Model file for the job. Use its own axes, mm. A direction names the side the tool comes from. Round coordinates to 2 decimals unless told otherwise and drop trailing zeros. Order: outer loops, then holes, each group sorted by start corner. A loop starts at its lowest first (then second) coordinate and runs counter-clockwise, first axis right, second up. Notation, with made-up numbers: (32.5, 4.25) -> (37.5, 4.25) arc R22 cw to (37.5, 40.25) -> close; hole circle Ø10 at (34, 46). An arc over 180 degrees is marked (long way). Answer as CSV lines item,"result".
```python
from build123d import *

# Parameters (mm, degrees)
F1_DEPTH     = 3.175
F3_W         = 1562.1
F3_H         = 50.8
F4_DEPTH     = 3.175
F5_T         = 2.54
F5_T3_DEPTH  = 8.255
F5_T5_DEPTH  = 1567.18
F6_T         = 2.54
F6_T3_DEPTH  = 8.255
F6_T5_DEPTH  = 8.255
F6_T7_DEPTH  = 1567.18
F6_T9_DEPTH  = 5.715
F6_T11_DEPTH = 50.165
F6_T13_DEPTH = 5.715
F6_T15_DEPTH = 1562.1


# Not quite as in the source:
# - a shell that OpenCascade refuses in one call is made with other operations: the cavity is built on its own and cut out


with BuildPart() as f1:
    # F0 (on Front) → F1 (new body)
    with BuildSketch(Plane.XZ):
        Polygon((-781.05, 156.1854919385), (-793.75, 156.1854919385), (-793.75, 3.7854919385), (793.75, 3.7854919385), (793.75, 156.1854919385), (781.05, 156.1854919385), (781.05, 35.5354919385), (-781.05, 35.5354919385), align=None)
    extrude(amount=F1_DEPTH)

    # F3 (on face) → F4 (join)
    with BuildSketch(Plane.XY.offset(35.5354919385)):
        with Locations((0, 22.225)):
            Rectangle(F3_W, F3_H)
    extrude(amount=-F4_DEPTH)

    # F5: shell of thickness 2.54, made by hand


with BuildPart() as f5_core1:
    # F5_t2: copy of F1
    add(f1.part)

    # the walls: a layer under each face that stays
    f5_faces = [f5_core1.faces().sort_by_distance(p)[0] for p in [
        (-781.05, -1.5875, 95.8604919385),
        (-787.4, -1.5875, 156.1854919385),
        (-529.1666666667, 0, 29.1854919385),
        (-529.1666666667, -3.175, 29.1854919385),
        (781.05, -1.5875, 95.8604919385),
        (-793.75, -1.5875, 79.9854919385),
        (-781.05, 23.8125, 33.9479919385),
        (0, 23.8125, 32.3604919385),
        (781.05, 23.8125, 33.9479919385),
        (787.4, -1.5875, 156.1854919385),
        (793.75, -1.5875, 79.9854919385),
        (0, -1.5875, 3.7854919385),
        (0, 47.625, 33.9479919385),
    ]]
    thicken(f5_faces, amount=-F5_T, mode=Mode.SUBTRACT)

    # F5_s4 → F5_t3 (cut)
    with BuildSketch(Plane.XY.offset(29.8204919385)):
        Polygon((-781.0754, 0.0254), (-781.05, -2.54), (-778.51, -2.54), (-778.51, 0), align=None)
        Polygon((781.0754, 0.0254), (781.05, -2.54), (778.51, -2.54), (778.51, 0), align=None)
    extrude(amount=F5_T3_DEPTH, mode=Mode.SUBTRACT)

    # F5_s6 → F5_t5 (cut)
    with BuildSketch(Plane.YZ.offset(-783.59)):
        Polygon((0.0254, 32.3350919385), (-2.54, 32.3604919385), (-2.54, 34.9004919385), (0, 34.9004919385), align=None)
    extrude(amount=F5_T5_DEPTH, mode=Mode.SUBTRACT)


with BuildPart() as f1_1:
    add(f1.part)

    # what is left inside the walls is the cavity
    f5_cavity = [f5_core1.part.solids().sort_by_distance(p)[0] for p in [
        (0, 14.605, 34.925892),
    ]]
    add(f5_cavity, mode=Mode.SUBTRACT)

    # F6: shell of thickness 2.54, made by hand


with BuildPart() as f6_core1:
    # F6_t2: copy of F1
    add(f1_1.part)

    # the walls: a layer under each face that stays
    f6_faces = [f6_core1.faces().sort_by_distance(p)[0] for p in [
        (-781.05, -1.5875, 95.8604919385),
        (728.98, -1.4816666667, 35.5354919385),
        (-787.4, -1.5875, 156.1854919385),
        (-529.1666666667, 0, 29.1854919385),
        (781.05, -1.5875, 95.8604919385),
        (781.05, 23.8125, 33.9479919385),
        (0, 47.625, 33.9479919385),
        (-781.05, 23.8125, 33.9479919385),
        (778.51, 22.225, 35.2179919385),
        (0, -0.635, 35.2179919385),
        (-778.51, 22.225, 35.2179919385),
        (0, 45.085, 35.2179919385),
        (-793.75, -1.5875, 79.9854919385),
        (0, 23.8125, 32.3604919385),
        (787.4, -1.5875, 156.1854919385),
        (793.75, -1.5875, 79.9854919385),
        (0, -1.5875, 3.7854919385),
        (0, 22.225, 34.9004919385),
    ]]
    thicken(f6_faces, amount=-F6_T, mode=Mode.SUBTRACT)

    # F6_s4 → F6_t3 (cut)
    with BuildSketch(Plane.XZ.offset(-2.54)):
        Polygon((-781.0246, 35.5608919385), (-783.59, 35.5354919385), (-783.59, 32.9954919385), (-781.05, 32.9954919385), align=None)
        Polygon((781.0246, 35.5608919385), (781.05, 32.9954919385), (783.59, 32.9954919385), (783.59, 35.5354919385), align=None)
    extrude(amount=F6_T3_DEPTH, mode=Mode.SUBTRACT)

    # F6_s6 → F6_t5 (cut)
    with BuildSketch(Plane.XY.offset(29.8204919385)):
        Polygon((-781.0754, 0.0254), (-781.05, -2.54), (-778.51, -2.54), (-778.51, 0), align=None)
        Polygon((781.0754, 0.0254), (781.05, -2.54), (778.51, -2.54), (778.51, 0), align=None)
    extrude(amount=F6_T5_DEPTH, mode=Mode.SUBTRACT)

    # F6_s8 → F6_t7 (cut)
    with BuildSketch(Plane.YZ.offset(-783.59)):
        Polygon((0.0254, 32.3350919385), (-2.54, 32.3604919385), (-2.54, 34.9004919385), (0, 34.9004919385), align=None)
    extrude(amount=F6_T7_DEPTH, mode=Mode.SUBTRACT)

    # F6_s10 → F6_t9 (cut)
    with BuildSketch(Plane.XY.offset(32.3604919385)):
        Polygon((778.4846, 45.0596), (781.05, 45.085), (781.05, 47.625), (778.51, 47.625), align=None)
        Polygon((778.4846, -0.6096), (781.05, -0.635), (781.05, -3.175), (778.51, -3.175), align=None)
        Polygon((-778.4846, -0.6096), (-778.51, -3.175), (-781.05, -3.175), (-781.05, -0.635), align=None)
        Polygon((-778.4846, 45.0596), (-781.05, 45.085), (-781.05, 47.625), (-778.51, 47.625), align=None)
    extrude(amount=F6_T9_DEPTH, mode=Mode.SUBTRACT)

    # F6_s12 → F6_t11 (cut)
    with BuildSketch(Plane.XZ.offset(-47.625)):
        Polygon((778.4846, 34.9258919385), (781.05, 34.9004919385), (781.05, 32.3604919385), (778.51, 32.3604919385), align=None)
        Polygon((-778.4846, 34.9258919385), (-781.05, 34.9004919385), (-781.05, 32.3604919385), (-778.51, 32.3604919385), align=None)
    extrude(amount=F6_T11_DEPTH, mode=Mode.SUBTRACT)

    # F6_s14 → F6_t13 (cut)
    with BuildSketch(Plane.XZ.offset(-2.54)):
        Polygon((778.4846, 34.9258919385), (781.05, 34.9004919385), (781.05, 32.3604919385), (778.51, 32.3604919385), align=None)
        Polygon((-778.4846, 34.9258919385), (-781.05, 34.9004919385), (-781.05, 32.3604919385), (-778.51, 32.3604919385), align=None)
    extrude(amount=F6_T13_DEPTH, mode=Mode.SUBTRACT)

    # F6_s16 → F6_t15 (cut)
    with BuildSketch(Plane.YZ.offset(-781.05)):
        Polygon((-0.6096, 34.9258919385), (-3.175, 34.9004919385), (-3.175, 32.3604919385), (-0.635, 32.3604919385), align=None)
        Polygon((45.0596, 34.9258919385), (47.625, 34.9004919385), (47.625, 32.3604919385), (45.085, 32.3604919385), align=None)
    extrude(amount=F6_T15_DEPTH, mode=Mode.SUBTRACT)


with BuildPart() as f1_2:
    add(f1_1.part)

    # what is left inside the walls is the cavity
    f6_cavity = [f6_core1.part.solids().sort_by_distance(p)[0] for p in [
        (395.605, -2.5654, 22.694381),
    ]]
    add(f6_cavity, mode=Mode.SUBTRACT)


solid = f1_2.part
```
Q1. Flat gauge pins, fed straight in: pin 1 (3 mm diameter, centred on x = -313, y = 5.5, fed in from +Z); pin 2 (1.6 mm diameter, centred on y = 14.5, z = 33.5, fed in from +X); pin 3 (0.5 mm diameter, centred on x = -103, y = -3, fed in from +Z). Where does each tip first touch, or does it go through?
Checks:
pin 1,"z = 34.9"
pin 2,"x = 781.05"
pin 3,"z = 35.54"
Q2. Saw through at C-C (x = 440). Write the cut outline in (y, z) (1 decimal).
Checks:
outline,"(-3.2, 3.8) -> (0, 3.8) -> (0, 32.4) -> (47.6, 32.4) -> (47.6, 35.5) -> (45.1, 35.5) -> (45.1, 34.9) -> (-0.6, 34.9) -> (-0.6, 35.5) -> (-3.2, 35.5) -> (-3.2, 32.4) -> (-2.5, 32.4) -> (-2.5, 6.3) -> (-3.2, 6.3) -> close"
Q3. Wall check: L1, parallel to Z at x = -432, y = 21. Give the ranges that are in metal, low to high. Write a range as [from, to].
Checks:
L1,"[32.36, 34.9]"
Q4. Tool access for faces 1 (the flat face through (-11, 24, 32.36)), 2 (the flat face through (4, -2, 35.535)), 3 (the flat face through (-4, -3.175, 35)): list every direction of +Z, -Z, +X, -X, +Y, -Y with a clear straight run to the whole face (end or side of a thin tool).
Checks:
face 1,"-Z, +X, -X, +Y"
face 2,"+Z, +Y, -Y"
face 3,"+Z, -Z, +X, -X, -Y"
Q5. Saw through at A-A (z = 106). Write the cut outline in (x, y) (3 decimals).
Checks:
outline,"(-793.75, -3.175) -> (-791.21, -3.175) -> (-791.21, -2.54) -> (-783.59, -2.54) -> (-783.59, -3.175) -> (-781.05, -3.175) -> (-781.05, 0) -> (-793.75, 0) -> close; (781.05, -3.175) -> (783.59, -3.175) -> (783.59, -2.54) -> (791.21, -2.54) -> (791.21, -3.175) -> (793.75, -3.175) -> (793.75, 0) -> (781.05, 0) -> close"
Q6. Saw through at B-B (y = 8.5). Write the cut outline in (x, z), plus the area to 3 significant figures.
Checks:
outline,"(-781.05, 32.36) -> (781.05, 32.36) -> (781.05, 35.54) -> (778.51, 35.54) -> (778.51, 34.9) -> (-778.51, 34.9) -> (-778.51, 35.54) -> (-781.05, 35.54) -> close"
area,"3,970 mm²"
